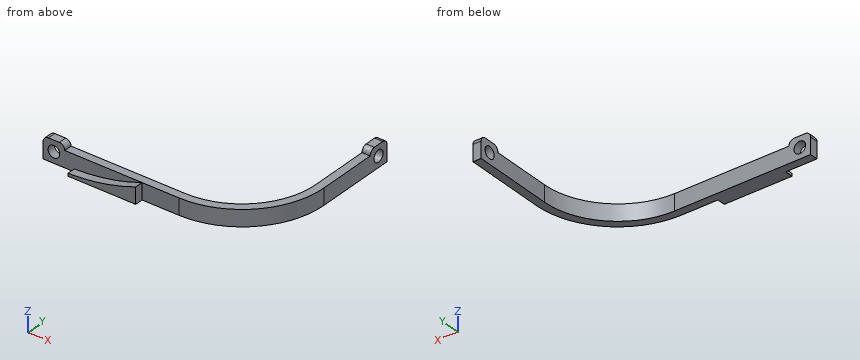
Autodesk Inventor part; units mm, degrees
ref_plane "YZ Plane" through (0, 0, 0) normal (1, 0, 0) x (0, 1, 0)
ref_plane "XZ Plane" through (0, 0, 0) normal (0, 1, 0) x (-1, 0, 0)
ref_plane "XY Plane" through (0, 0, 0) normal (0, 0, 1) x (1, 0, 0)
sketch "Sketch1" plane through (0, 0, 0) normal (0, 0, 1) x (1, 0, 0)
  line L0 (0, 0) -> (60, 0) construction
  line L1 (60, 0) -> (60, 60) construction
  line L2 (60, 60) -> (0, 60) construction
  line L3 (0, 3) -> (0, 0)
  line L4 (57, 60) -> (60, 60)
  line L5 (60, 60) -> (60, 30)
  line L6 (60, 0) -> (30, 0) construction
  line L7 (30, 0) -> (30, 30) construction
  line L8 (30, 30) -> (60, 30) construction
  line L9 (60, 30) -> (60, 0) construction
  arc A0 (30, 3) -> (57, 30) centre (30, 30) ccw
  line L10 (30, 3) -> (0, 3)
  line L11 (0, 0) -> (30, 0)
  line L12 (57, 30) -> (57, 60)
  line L13 (0, 60) -> (0, 30) construction
  line L14 (0, 3) -> (0, 0) construction
  arc A1 (30, 0) -> (60, 30) centre (30, 30) ccw
  arc A2 (30, 60) -> (0, 30) centre (30, 30) ccw
  dimension "d0" = 60
  dimension "d1" = 60
  dimension "d3" = 3
  dimension "d6" = 30
extrude "Extrusion2" add sketch "Sketch1" along normal blind 6
sketch "Sketch4" plane through (0, 0, 6) normal (0, 0, 1) x (1, 0, 0)
  line L0 (60, 30) -> (60, 60)
  line L1 (57, 60) -> (60, 60)
  line L2 (60, 60) -> (60, 52)
  line L3 (60, 52) -> (57, 52)
  line L4 (57, 52) -> (57, 60)
  point P0 (0, 0)
  dimension "d16" = 8
extrude "Extrusion5" add sketch "Sketch4" along normal blind 2
sketch "Sketch5" plane through (57, 30, 0) normal (-1, 0, 0) x (0, 0, 1)
  circle A0 centre (4, 26) radius 2.15
  point P0 (0, -30)
  dimension "d19" = 4.3
extrude "Extrusion6" cut sketch "Sketch5" against normal through all
fillet "Fillet1" radius 2 2 edges at (58.5, 52, 8) (58.5, 60, 8)
sketch "Sketch8" plane through (0, 0, 0) normal (0, 0, 1) x (1, 0, 0)
  line L0 (0, 0) -> (-20, 0)
  line L1 (-20, 0) -> (-20, 3)
  line L2 (-20, 3) -> (0, 3)
  line L3 (0, 3) -> (0, 0)
  dimension "d32" = 20
  dimension "d33" = 3
extrude "Extrusion9" add sketch "Sketch8" along normal blind 6
sketch "Sketch9" plane through (0, 0, 6) normal (0, 0, 1) x (1, 0, 0)
  line L0 (-20, 3) -> (-20, 0)
  line L1 (-20, 0) -> (-12, 0)
  line L2 (-12, 0) -> (-12, 3)
  line L3 (-12, 3) -> (-20, 3)
  line L4 (-20, 3) -> (-20, 0)
  dimension "d36" = 8
extrude "Extrusion10" add sketch "Sketch9" along normal blind 2
sketch "Sketch11" plane through (30, 0, 0) normal (0, -1, 0) x (1, 0, 0)
  circle A0 centre (-46, 4) radius 2.15
  point P0 (-30, 0)
  dimension "d43" = 4.3
extrude "Extrusion12" cut sketch "Sketch11" against normal through all
fillet "Fillet3" radius 2 2 edges at (-20, 1.5, 8) (-12, 1.5, 8)
sketch "Sketch12" plane through (30, 0, 0) normal (0, -1, 0) x (1, 0, 0)
  line L0 (-48, 8) -> (-44, 8)
  line L1 (0, 0) -> (-50, 0)
  line L2 (0, 0) -> (0, 6)
  line L3 (-42, 6) -> (0, 6)
  arc A0 (-38.5519, 1.0253) -> (34.1434, 68.6948) centre (-40.5, 76) ccw
  line L4 (-38.474, 1.0274) -> (-38.474, 0)
  line L5 (-13.5742, 6) -> (-13.5742, 2.7948)
  arc A1 (-38.5519, 1.0253) -> (34.1434, 68.6948) centre (-40.5, 76) ccw
  arc A2 (-2.2901, 8) -> (37.1291, 68.4026) centre (-40.5, 76) ccw
  line L6 (-30.8178, 0) -> (-22.9501, 0)
  line L7 (-13.5742, 2.7948) -> (-13.5742, 6)
  line L8 (-13.5742, 2.4368) -> (-13.5742, 6)
  arc A3 (-38.474, 1.0274) -> (-13.5742, 6) centre (-40.5, 76) ccw
  line L9 (-38.474, 0) -> (-22.9501, 0)
  line L10 (-38.474, 1.2893) -> (-38.474, 0)
  line L11 (-19.033, 0) -> (-41.5355, 0)
  line L12 (-13.5742, 6) -> (-13.5742, 0)
  line L13 (-13.5742, 0) -> (-24.5114, 0)
  point P0 (-30, 0)
extrude "Extrusion13" add sketch "Sketch12" along normal blind 3
sketch "Sketch13" plane through (30, -3, 0) normal (0, -1, 0) x (1, 0, 0)
  line L0 (0, 0) -> (-13.5742, 0)
  line L1 (-13.5742, 0) -> (-13.5742, 6)
  line L2 (-13.5742, 6) -> (0, 6)
  line L3 (0, 6) -> (0, 0)
  point P0 (-30, 0)
extrude "Extrusion14" cut sketch "Sketch13" against normal blind 3
properties part number "FrontNetHook"
The model under review builds one solid part; all positions refer to its coordinate system, in mm. Coordinates: 2 decimals unless noted, no trailing zeros. Loops run counter-clockwise (first coordinate to the right, second up) from the corner with the lowest first, then second, coordinate; pieces in that order, holes last. Notation, with made-up numbers: M 34,50 L 52,50 A16 ccw 52,61 Z; hole C -19,84.5 d2. An arc over 180 degrees is marked long. Put each result on its own line as item: value. Start each with the question number.
Q1. Add section A-A (y = 56). Write out the cut boundary in (x, z).
Q2. Add section C-C (z = 3). Write out the cut boundary in (x, y), and give its area (3 significant figures).
Q3. Wall thickness on line 1 (Z direction, x = -16, y = 1.9); line 2 (Y direction, x = 23, z = 5.5); line 3 (X direction, y = 2.5, z = 5.5): over which ranges is each line inside the solid? List them lowest first.
Q4. Add section B-B (x = -16). Write out the cut boundary in (y, z), and give its area (3 significant figures).
Q5. Add section D-D (x = 24). Write out the cut boundary in (y, z), and give its area (3 significant figures).
Q6. Clearance check with flat-ended pins moving along their axes: pin 1 (3.5 mm diameter, centred on x = -16, z = 4, fed in from -Y); pin 2 (2 mm diameter, centred on x = -9.5, z = 6, fed in from -Y); pin 3 (3 mm diameter, centred on y = 23.5, z = 5, fed in from -X); pin 4 (2.5 mm diameter, centred on y = -2, z = 2.5, fed in from +X). State where each tip first meets the part, or that it passes through.
Answers:
1. outline: M 57,0 L 60,0 L 60,1.85 L 57,1.85 Z; M 57,6.15 L 60,6.15 L 60,8 L 57,8 Z
2. outline: M -20,0 L -17.9,0 L -17.9,3 L -20,3 Z; M -14.1,0 L 6.7,0 L 6.7,-3 L 16.43,-3 L 16.43,0 L 30,0 A30 ccw 60,30 L 60,54.1 L 57,54.1 L 57,30 A27 cw 30,3 L -14.1,3 Z; M 57,57.9 L 60,57.9 L 60,60 L 57,60 Z
2. area: 381 mm^2
3. line 1: z = 0 to 1.85, 6.15 to 8
3. line 2: y = 0 to 3
3. line 3: x = -20 to -17.54, -14.46 to 41.99
4. outline: M 0,0 L 3,0 L 3,1.85 L 0,1.85 Z; M 0,6.15 L 3,6.15 L 3,8 L 0,8 Z
4. area: 11.1 mm^2
5. outline: M 0,0 L 3,0 L 3,6 L 0,6 Z
5. area: 18.0 mm^2
6. pin 1: passes through
6. pin 2: stops at y = 0
6. pin 3: stops at x = 55.79
6. pin 4: stops at x = 16.43
